Build history of the part. All positions in model axes, mm. Face numbers are marked on the shaded views. A direction names the side the tool comes from. Give positions to 0.01 mm unless a question says otherwise; leave off trailing zeros. Loops run counter-clockwise (first coordinate to the right, second up) from the corner with the lowest first, then second, coordinate; pieces in that order, holes last. Notation, with made-up numbers: (23.5, 40) -> (37.5, 40) arc R20 ccw to (37.5, 72) -> close; hole circle Ø6 at (56.5, 39). An arc over 180 degrees is marked (long way). Answer in a Markdown table with one row per item. Add a question column.
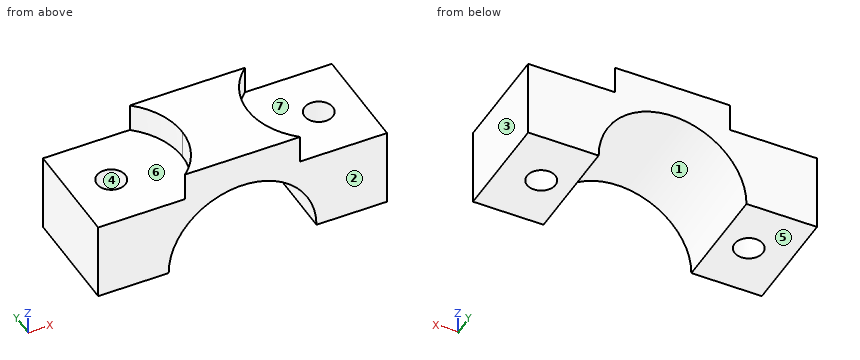
from build123d import *

# Parameters (mm, degrees)
SKETCH2_W               = 50.8
SKETCH2_H               = 19
BOSS_EXTRUDE1_DEPTH     = 19
SKETCH3_R               = 13
CUT_EXTRUDE1_DEPTH      = 20
SKETCH4_R               = 2.5
CUT_EXTRUDE2_DEPTH      = 5
SKETCH5_R               = 2.5
CUT_EXTRUDE3_DEPTH      = 1
CUT_EXTRUDE3_DEPTH_BACK = 20


with BuildPart() as part:
    # Sketch2 → Boss-Extrude1 (new body)
    with BuildSketch(Plane.XY):
        Rectangle(SKETCH2_W, SKETCH2_H)
    extrude(amount=BOSS_EXTRUDE1_DEPTH)

    # Sketch3 → Cut-Extrude1 (cut, through all)
    with BuildSketch(Plane.XZ.offset(9.5)):
        Circle(SKETCH3_R)
    extrude(amount=-CUT_EXTRUDE1_DEPTH, mode=Mode.SUBTRACT)

    # Sketch4 → Cut-Extrude2 (cut)
    with BuildSketch(Plane.XY.offset(19)):
        with BuildLine():
            ThreePointArc((-10.125961595, -9.5), (-6.896575846, -5.229699797), (-5.75, 0))
            ThreePointArc((-5.75, 0), (-6.896575846, 5.229699797), (-10.125961595, 9.5))
            Line((-10.125961595, 9.5), (-25.4, 9.5))
            Line((-25.4, 9.5), (-25.4, -9.5))
            Line((-25.4, -9.5), (-10.125961595, -9.5))
        make_face()
        with Locations((-18.25, 0)):
            Circle(SKETCH4_R, mode=Mode.SUBTRACT)
        with BuildLine():
            Line((25.4, 9.5), (10.125961595, 9.5))
            ThreePointArc((10.125961595, 9.5), (5.75, 0), (10.125961595, -9.5))
            Line((10.125961595, -9.5), (25.4, -9.5))
            Line((25.4, -9.5), (25.4, 9.5))
        make_face()
        with Locations((18.25, 0)):
            Circle(SKETCH4_R, mode=Mode.SUBTRACT)
    extrude(amount=-CUT_EXTRUDE2_DEPTH, mode=Mode.SUBTRACT)

    # Sketch5 → Cut-Extrude3 (cut, two sides)
    with BuildSketch(Plane.XY.offset(19)) as cut_extrude3_sk:
        with Locations((18.25, 0)):
            Circle(SKETCH5_R)
        with Locations((-18.25, 0)):
            Circle(SKETCH5_R)
    extrude(amount=CUT_EXTRUDE3_DEPTH, mode=Mode.SUBTRACT)
    extrude(cut_extrude3_sk.sketch, amount=-CUT_EXTRUDE3_DEPTH_BACK, mode=Mode.SUBTRACT)


solid = part.part
(1) 3-axis set-ups, long thin cutter, end or side, ignore diameter. For the marked faces 5, 6 and 7: which of +Z, -Z, +X, -X, +Y, -Y reach the whole face in a straight line?
(2) Saw through at D-D, the plane z = 6. List the corners of the cut face in (x, y).
(3) Flat gauge pins, fed straight in: pin 1 Ø5 at (x, y) = (18.5, 1.5) entering from +Z; pin 2 Ø4.5 at (x, y) = (18.25, 0) entering from -Z. Where does each tip first touch, or does it go through?
(4) Saw through at B-B, the plane z = 8.5. List the corners of the cut face in (x, y).
(5) Saw through at C-C, the plane y = -1.5. List the corners of the cut face in (x, z), then the cut area to 3 significant figures.
(6) Wall check: line 1 along Y through (x, z) = (18.25, 5.5); line 2 along Z through (x, y) = (22.5, 4.5); line 3 along Y through (x, z) = (-19, 11.75). Give the ranges that are in metal, low to high. Write a range as from..to.
(7) Saw through at A-A, the plane x = 18.25. List the corners of the cut face in (y, z).
(8) Two-plate mould, pull along X, no slides. Class the marked faces 1, 2, 3 and 4: released by +X, released by -X, zero draft, split by the parting line, or undercut.
Worked answers:
| question | item | result |
|---|---|---|
| 1 | face 5 | -Z, +X, -X, +Y, -Y |
| 1 | face 6 | +Z, -X |
| 1 | face 7 | +Z, +X |
| 2 | outline | (-25.4, -9.5) -> (-11.53, -9.5) -> (-11.53, 9.5) -> (-25.4, 9.5) -> close; (11.53, -9.5) -> (25.4, -9.5) -> (25.4, 9.5) -> (11.53, 9.5) -> close; hole circle Ø5 at (-18.25, 0); hole circle Ø5 at (18.25, 0) |
| 3 | pin 1 | z = 14 |
| 3 | pin 2 | through |
| 4 | outline | (-25.4, -9.5) -> (-9.84, -9.5) -> (-9.84, 9.5) -> (-25.4, 9.5) -> close; (9.84, -9.5) -> (25.4, -9.5) -> (25.4, 9.5) -> (9.84, 9.5) -> close; hole circle Ø5 at (-18.25, 0); hole circle Ø5 at (18.25, 0) |
| 5 | outline | (-25.4, 0) -> (-20.25, 0) -> (-20.25, 14) -> (-25.4, 14) -> close; (-16.25, 0) -> (-13, 0) arc R13 cw to (13, 0) -> (16.25, 0) -> (16.25, 14) -> (5.84, 14) -> (5.84, 19) -> (-5.84, 19) -> (-5.84, 14) -> (-16.25, 14) -> close; (20.25, 0) -> (25.4, 0) -> (25.4, 14) -> (20.25, 14) -> close |
| 5 | area | 392 mm^2 |
| 6 | line 1 | -9.5..-2.5, 2.5..9.5 |
| 6 | line 2 | 0..14 |
| 6 | line 3 | -9.5..-2.38, 2.38..9.5 |
| 7 | outline | (-9.5, 0) -> (-2.5, 0) -> (-2.5, 14) -> (-9.5, 14) -> close; (2.5, 0) -> (9.5, 0) -> (9.5, 14) -> (2.5, 14) -> close |
| 8 | face 1 | undercut |
| 8 | face 2 | zero draft |
| 8 | face 3 | released by +X |
| 8 | face 4 | undercut |
